Design review of the part shown in the three views and the two pictorial views. Dimensions are in mm from the part's minimum x, y and z. A direction names the side the tool comes from. Give positions to 0.01 mm unless a question says otherwise; leave off trailing zeros. Write each loop counter-clockwise with the first axis right and the second up, starting at its lowest first coordinate (ties: lowest second). Pieces come first, ordered by that corner, then holes. Notation, with made-up numbers: M 50.5,30.25 L 54.5,30.25 A22 cw 54.5,52.25 Z; hole C 21.25,-7 d10. An arc over 180 degrees is marked long. Write item = value, one per line.
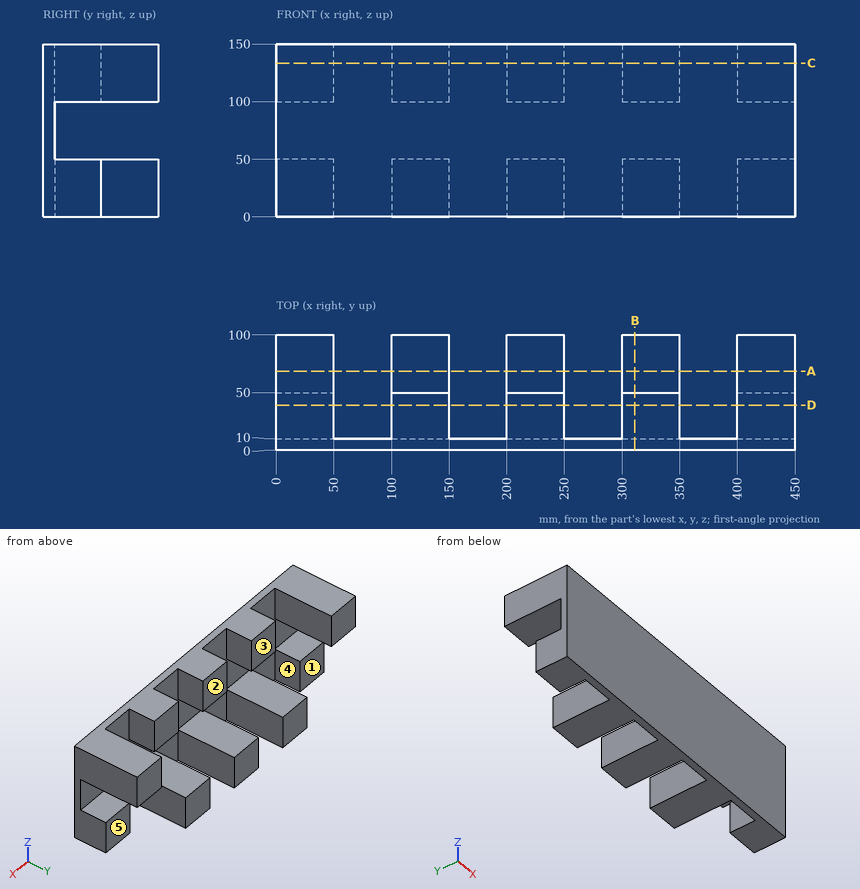
1. For line 1 along X through (y, z) = (60.5, 33); line 2 along X through (y, z) = (46.5, 115); line 3 along X through (y, z) = (92.5, 115), list the stretches that pass through material, from the lowest coordinate up. Write a range as from..to.
Responses:
line_1 = 100..150, 200..250, 300..350
line_2 = 0..50, 100..150, 200..250, 300..350, 400..450
line_3 = 0..50, 400..450
2. We need section B-B, the plane x = 311. Write out the cut boundary in (y, z), then the cut area to 3 significant figures.
Responses:
outline = M 0,0 L 100,0 L 100,50 L 10,50 L 10,100 L 50,100 L 50,150 L 0,150 Z
area = 8,000 mm2
3. Machinability: for the marked faces 3, 4 and 5, which of the approach directions +Z, -Z, +X, -X, +Y, -Y give a long, thin tool a straight path to every point of the face, cutting with its end or side? Answer none if there is none.
Responses:
face_3 = +Z, +Y
face_4 = +Z, -Z, +Y
face_5 = -Z, +X, +Y
4. Insertion check: P1, Ø6, axis at x = 190, z = 31, coming from the +Y side; P2, Ø25, axis at x = 131.5, z = 131.5, coming from the +Y side. Each pin has a flat end and moves straight along its axis. Give the tip position at first contact, or say it passes through.
Responses:
P1 = 10
P2 = 50
5. We need section D-D, the plane y = 39. Count the separate pieces of the cut face and the enclosed holes in it, then the cut area to 3 significant figures.
Responses:
separate_pieces = 10
enclosed_holes = 0
area = 25,000 mm2
6. We need section A-A, the plane y = 68.5. Write out the cut boundary in (x, z).
Responses:
outline = M 0,100 L 50,100 L 50,150 L 0,150 Z; M 100,0 L 150,0 L 150,50 L 100,50 Z; M 200,0 L 250,0 L 250,50 L 200,50 Z; M 300,0 L 350,0 L 350,50 L 300,50 Z; M 400,100 L 450,100 L 450,150 L 400,150 Z
7. We need section C-C, the plane z = 133.5. Write out the cut boundary in (x, y).
Responses:
outline = M 0,0 L 450,0 L 450,100 L 400,100 L 400,10 L 350,10 L 350,50 L 300,50 L 300,10 L 250,10 L 250,50 L 200,50 L 200,10 L 150,10 L 150,50 L 100,50 L 100,10 L 50,10 L 50,100 L 0,100 Z
8. The part is to be moulded in two halves that separate along X. For the marked faces 1 and 2, say which applies: +X half, -X half, draft (parallel to the pull), parting line (faces both ways), or undercut.
Responses:
face_1 = draft
face_2 = undercut
